Autodesk Inventor part; units mm, degrees
ref_plane "YZ Plane" through (0, 0, 0) normal (1, 0, 0) x (0, 1, 0)
ref_plane "XZ Plane" through (0, 0, 0) normal (0, 1, 0) x (-1, 0, 0)
ref_plane "XY Plane" through (0, 0, 0) normal (0, 0, 1) x (1, 0, 0)
sketch "Sketch1" plane through (0, 0, 0) normal (1, 0, 0) x (0, 1, 0)
  circle A0 centre (0, 0) radius 3.1
  arc A1 (0, 5) -> (0, -5) centre (0, 0) ccw
  line L0 (0, 5) -> (50, 5)
  line L1 (50, -5) -> (0, -5)
  arc A2 (50, -5) -> (50, 5) centre (50, 0) ccw
  circle A3 centre (50, 0) radius 3.1
  dimension "d0" = 6.2
  dimension "d1" = 10
  dimension "d3" = 50
  dimension "d5" = 6.2
  dimension "d26" = 5
extrude "Extrusion1" add sketch "Sketch1" along normal blind 3
ref_plane "Work Plane1" through (-2, 0, 0) normal (1, 0, 0) x (0, 0, -1)
sketch "Sketch5" plane through (3, 0, 0) normal (1, 0, 0) x (0, 0, -1)
  line L0 (-5, 50) -> (-5, 0)
  arc A0 (-5, 0) -> (5, 0) centre (0, 0) ccw
  circle A1 centre (0, 50) radius 3.1
  circle A2 centre (0, 0) radius 3.1
  arc A3 (-5, 0) -> (5, 0) centre (0, 0) ccw
  line L1 (5, 0) -> (5, 50)
  arc A4 (5, 50) -> (-5, 50) centre (0, 50) ccw
  line L2 (-5, 50) -> (-5, 0)
  line L3 (0, -5) -> (0, 6)
  line L4 (0, 6) -> (5, 11)
  line L5 (5, 0) -> (5, 50)
  line L6 (0, 6) -> (-5, 11)
  line L7 (0, 55) -> (0, 44)
  line L8 (0, 44) -> (-5, 39)
  line L9 (0, 44) -> (5, 39)
  line L10 (0, 44) -> (7.0711, 44) construction
  dimension "d27" = 11
  dimension "d28" = 135
  dimension "d29" = 11
  dimension "d30" = 135
  dimension "d31" = 45
equation "\"d5\" = d0"
equation "\"d26\" = 0.5 * d1"
equation "\"d29\" = d27"
equation "\"d30\" = d28"
properties part number "ArmSpan"
Can you work these out from the model? Positions are in its coordinate system, mm. Round coordinates to 2 decimals unless told otherwise and drop trailing zeros. Loops run counter-clockwise (first coordinate to the right, second up) from the corner with the lowest first, then second, coordinate; pieces in that order, holes last. Notation, with made-up numbers: M -4,-6 L 12,-6 A25 ccw 12,11 Z; hole C 22.25,-33 d6. An arc over 180 degrees is marked long. Answer in a Markdown table with one row per item.
1. If we section it at C-C, the plane z = -3.75: Please give me the cut outline in (x, y), plus the area to 3 significant figures.
Established:
| item | result |
|---|---|
| outline | M 0,-3.31 L 3,-3.31 L 3,53.31 L 0,53.31 Z |
| area | 170 mm² |
2. If we section it at A-A, the plane z = 0: Please give me the cut outline in (x, y).
Established:
| item | result |
|---|---|
| outline | M 0,-5 L 3,-5 L 3,-3.1 L 0,-3.1 Z; M 0,3.1 L 3,3.1 L 3,46.9 L 0,46.9 Z; M 0,53.1 L 3,53.1 L 3,55 L 0,55 Z |
3. Please list where these lines run through material, in increasing order: line 1 (Y direction, x = 1.95, z = -2.75); line 2 (Y direction, x = 2.4, z = -1); line 3 (Z direction, x = 2.1, y = 0). Write a range as from..to.
Established:
| item | result |
|---|---|
| line 1 | -4.18..-1.43, 1.43..48.57, 51.43..54.18 |
| line 2 | -4.9..-2.93, 2.93..47.07, 52.93..54.9 |
| line 3 | -5..-3.1, 3.1..5 |
4. If we section it at B-B, the plane x = 0.65: Please give me the cut outline in (y, z).
Established:
| item | result |
|---|---|
| outline | M 0,-5 L 50,-5 A5 ccw 50,5 L 0,5 A5 ccw Z; hole C 0,0 d6.2; hole C 50,0 d6.2 |
5. Thinking about a two-plate mould opening in Y: for faces 1 (the face through (1.479, 52.864, 1.187)), 2 (the face through (1, 55, 0)), 3 (the face through (1, 25, 5)), which applies, pulls with the +Y half, pulls with the -Y half, needs draft (parallel to the pull), parting line crosses it, or undercut?
Established:
| item | result |
|---|---|
| face 1 | undercut |
| face 2 | pulls with the +Y half |
| face 3 | needs draft |
